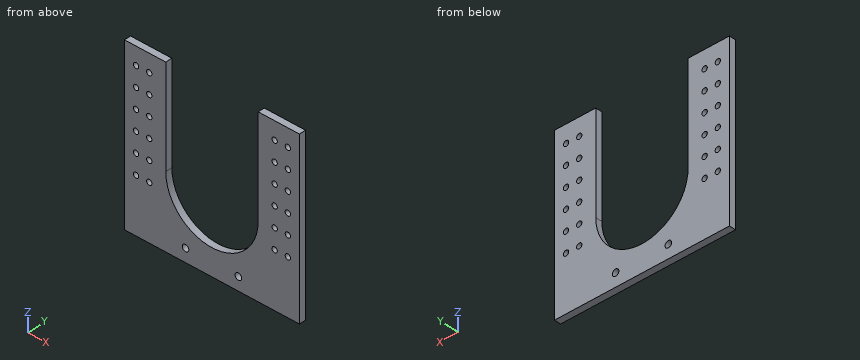
```python
from build123d import *

# Parameters (mm, degrees)
SKETCH1_W                        = 168.275
SKETCH1_H                        = 165.1
BOSS_EXTRUDE1_DEPTH              = 3.175
CUT_EXTRUDE1_REACH               = 120.042
SKETCH2_R                        = 44.45
F_1_4_0_25_DIAMETER_HOLE1_D      = 6.35
F_1_4_0_25_DIAMETER_HOLE1_DEPTH  = 25.4
F_1_4_0_25_DIAMETER_HOLE1_TIP    = 1.907732465
F_1_4_20_TAPPED_HOLE1_AT_2_COUNT = 2
F_1_4_20_TAPPED_HOLE1_AT_2_PITCH = 12.7
LPATTERN1_COUNT                  = 6
LPATTERN1_PITCH                  = 19.05


with BuildPart() as part:
    # Sketch1 → Boss-Extrude1 (new, symmetric)
    with BuildSketch(Plane(origin=(0, 0, 0), x_dir=(1, 0, 0), z_dir=(0, 1, 0))):
        Rectangle(SKETCH1_W, SKETCH1_H)
    extrude(amount=BOSS_EXTRUDE1_DEPTH, both=True)

    # Sketch2 → Cut-Extrude1 (cut, up to next)
    with BuildSketch(Plane(origin=(0, 3.175, 0), x_dir=(1, 0, 0), z_dir=(0, 1, 0)), mode=Mode.PRIVATE) as cut_extrude1_sk1:
        with Locations((0, 12.7)):
            Circle(SKETCH2_R)
    cut_extrude1_tool1 = extrude(cut_extrude1_sk1.sketch, amount=-CUT_EXTRUDE1_REACH, mode=Mode.PRIVATE) & part.part
    # Sketch2 → Cut-Extrude1 (cut, up to next)
    with BuildSketch(Plane(origin=(0, 3.175, 0), x_dir=(1, 0, 0), z_dir=(0, 1, 0)), mode=Mode.PRIVATE) as cut_extrude1_sk2:
        with BuildLine():
            Line((44.45, -82.55), (44.45, 12.7))
            ThreePointArc((44.45, 12.7), (0, -31.75), (-44.45, 12.7))
            Line((-44.45, 12.7), (-44.45, -82.55))
            Line((-44.45, -82.55), (44.45, -82.55))
        make_face()
    cut_extrude1_tool2 = extrude(cut_extrude1_sk2.sketch, amount=-CUT_EXTRUDE1_REACH, mode=Mode.PRIVATE) & part.part
    add(cut_extrude1_tool1.solids().sort_by_distance((0, 3.175, -12.7))[0], mode=Mode.SUBTRACT)
    add(cut_extrude1_tool2.solids().sort_by_distance((0, 3.175, 51.564855))[0], mode=Mode.SUBTRACT)

    # 1/4 (0.25) Diameter Hole1
    with Locations(Plane(origin=(0, 3.175, 0), x_dir=(1, 0, 0), z_dir=(0, 1, 0))):
        with Locations((-25.4, 69.85), (25.4, 69.85)):
            Hole(F_1_4_0_25_DIAMETER_HOLE1_D / 2, depth=F_1_4_0_25_DIAMETER_HOLE1_DEPTH)
            with Locations((0, 0, -(F_1_4_0_25_DIAMETER_HOLE1_DEPTH + F_1_4_0_25_DIAMETER_HOLE1_TIP / 2))):  # 118° drill point
                Cone(0, F_1_4_0_25_DIAMETER_HOLE1_D / 2, F_1_4_0_25_DIAMETER_HOLE1_TIP, mode=Mode.SUBTRACT)

    # Sketch10 → 1/4-20 Tapped Hole1 (revolve, cut)
    with BuildSketch(Plane(origin=(-73.025, 3.175, 65.603705108), x_dir=(0, 0, 1), z_dir=(1, 0, 0))):
        Polygon((0, 0), (0, 26.933816902), (2.5527, 25.4), (2.5527, 0), align=None)
    f_1_4_20_tapped_hole1 = revolve(axis=Axis((-73.025, 9.525, 65.603705108), (0, -1, 0)), mode=Mode.SUBTRACT)

    # 1/4-20 Tapped Hole1 at 2: 1/4-20 Tapped Hole1 ×2
    with Locations(*[(i * F_1_4_20_TAPPED_HOLE1_AT_2_PITCH, 0, 0) for i in range(1, F_1_4_20_TAPPED_HOLE1_AT_2_COUNT)]):
        add(f_1_4_20_tapped_hole1, mode=Mode.SUBTRACT)

    # LPattern1: 1/4-20 Tapped Hole1 ×6
    with Locations(*[(0, 0, -i * LPATTERN1_PITCH) for i in range(1, LPATTERN1_COUNT)]):
        add(f_1_4_20_tapped_hole1, mode=Mode.SUBTRACT)

    # LPattern1 copy 1 sketch → LPattern1 copy 1 (revolve, cut)
    with BuildSketch(Plane(origin=(-60.325, 3.175, 46.553705108), x_dir=(0, 0, 1), z_dir=(1, 0, 0))):
        Polygon((0, 0), (0, 26.933816902), (2.5527, 25.4), (2.5527, 0), align=None)
    revolve(axis=Axis((-60.325, 9.525, 46.553705108), (0, -1, 0)), mode=Mode.SUBTRACT)

    # LPattern1 copy 2 sketch → LPattern1 copy 2 (revolve, cut)
    with BuildSketch(Plane(origin=(-60.325, 3.175, 27.503705108), x_dir=(0, 0, 1), z_dir=(1, 0, 0))):
        Polygon((0, 0), (0, 26.933816902), (2.5527, 25.4), (2.5527, 0), align=None)
    revolve(axis=Axis((-60.325, 9.525, 27.503705108), (0, -1, 0)), mode=Mode.SUBTRACT)

    # LPattern1 copy 3 sketch → LPattern1 copy 3 (revolve, cut)
    with BuildSketch(Plane(origin=(-60.325, 3.175, 8.453705108), x_dir=(0, 0, 1), z_dir=(1, 0, 0))):
        Polygon((0, 0), (0, 26.933816902), (2.5527, 25.4), (2.5527, 0), align=None)
    revolve(axis=Axis((-60.325, 9.525, 8.453705108), (0, -1, 0)), mode=Mode.SUBTRACT)

    # LPattern1 copy 4 sketch → LPattern1 copy 4 (revolve, cut)
    with BuildSketch(Plane(origin=(-60.325, 3.175, -10.596294892), x_dir=(0, 0, 1), z_dir=(1, 0, 0))):
        Polygon((0, 0), (0, 26.933816902), (2.5527, 25.4), (2.5527, 0), align=None)
    revolve(axis=Axis((-60.325, 9.525, -10.596294892), (0, -1, 0)), mode=Mode.SUBTRACT)

    # LPattern1 copy 5 sketch → LPattern1 copy 5 (revolve, cut)
    with BuildSketch(Plane(origin=(-60.325, 3.175, -29.646294892), x_dir=(0, 0, 1), z_dir=(1, 0, 0))):
        Polygon((0, 0), (0, 26.933816902), (2.5527, 25.4), (2.5527, 0), align=None)
    revolve(axis=Axis((-60.325, 9.525, -29.646294892), (0, -1, 0)), mode=Mode.SUBTRACT)

    # Mirror1: 1/4-20 Tapped Hole1 across plane
    add(f_1_4_20_tapped_hole1.mirror(Plane(origin=(0, 0, 0), x_dir=(0, 0, 1), z_dir=(1, 0, 0))), mode=Mode.SUBTRACT)

    # Mirror1 copy 1 sketch → Mirror1 copy 1 (revolve, cut)
    with BuildSketch(Plane(origin=(60.325, 3.175, 65.603705108), x_dir=(0, 0, 1), z_dir=(-1, 0, 0))):
        Polygon((0, 0), (0, -26.933816902), (2.5527, -25.4), (2.5527, 0), align=None)
    revolve(axis=Axis((60.325, 9.525, 65.603705108), (0, 1, 0)), mode=Mode.SUBTRACT)

    # Mirror1 copy 2 sketch → Mirror1 copy 2 (revolve, cut)
    with BuildSketch(Plane(origin=(73.025, 3.175, 46.553705108), x_dir=(0, 0, 1), z_dir=(-1, 0, 0))):
        Polygon((0, 0), (0, -26.933816902), (2.5527, -25.4), (2.5527, 0), align=None)
    revolve(axis=Axis((73.025, 9.525, 46.553705108), (0, 1, 0)), mode=Mode.SUBTRACT)

    # Mirror1 copy 3 sketch → Mirror1 copy 3 (revolve, cut)
    with BuildSketch(Plane(origin=(73.025, 3.175, 27.503705108), x_dir=(0, 0, 1), z_dir=(-1, 0, 0))):
        Polygon((0, 0), (0, -26.933816902), (2.5527, -25.4), (2.5527, 0), align=None)
    revolve(axis=Axis((73.025, 9.525, 27.503705108), (0, 1, 0)), mode=Mode.SUBTRACT)

    # Mirror1 copy 4 sketch → Mirror1 copy 4 (revolve, cut)
    with BuildSketch(Plane(origin=(73.025, 3.175, 8.453705108), x_dir=(0, 0, 1), z_dir=(-1, 0, 0))):
        Polygon((0, 0), (0, -26.933816902), (2.5527, -25.4), (2.5527, 0), align=None)
    revolve(axis=Axis((73.025, 9.525, 8.453705108), (0, 1, 0)), mode=Mode.SUBTRACT)

    # Mirror1 copy 5 sketch → Mirror1 copy 5 (revolve, cut)
    with BuildSketch(Plane(origin=(73.025, 3.175, -10.596294892), x_dir=(0, 0, 1), z_dir=(-1, 0, 0))):
        Polygon((0, 0), (0, -26.933816902), (2.5527, -25.4), (2.5527, 0), align=None)
    revolve(axis=Axis((73.025, 9.525, -10.596294892), (0, 1, 0)), mode=Mode.SUBTRACT)

    # Mirror1 copy 6 sketch → Mirror1 copy 6 (revolve, cut)
    with BuildSketch(Plane(origin=(73.025, 3.175, -29.646294892), x_dir=(0, 0, 1), z_dir=(-1, 0, 0))):
        Polygon((0, 0), (0, -26.933816902), (2.5527, -25.4), (2.5527, 0), align=None)
    revolve(axis=Axis((73.025, 9.525, -29.646294892), (0, 1, 0)), mode=Mode.SUBTRACT)

    # Mirror1 copy 7 sketch → Mirror1 copy 7 (revolve, cut)
    with BuildSketch(Plane(origin=(60.325, 3.175, 46.553705108), x_dir=(0, 0, 1), z_dir=(-1, 0, 0))):
        Polygon((0, 0), (0, -26.933816902), (2.5527, -25.4), (2.5527, 0), align=None)
    revolve(axis=Axis((60.325, 9.525, 46.553705108), (0, 1, 0)), mode=Mode.SUBTRACT)

    # Mirror1 copy 8 sketch → Mirror1 copy 8 (revolve, cut)
    with BuildSketch(Plane(origin=(60.325, 3.175, 27.503705108), x_dir=(0, 0, 1), z_dir=(-1, 0, 0))):
        Polygon((0, 0), (0, -26.933816902), (2.5527, -25.4), (2.5527, 0), align=None)
    revolve(axis=Axis((60.325, 9.525, 27.503705108), (0, 1, 0)), mode=Mode.SUBTRACT)

    # Mirror1 copy 9 sketch → Mirror1 copy 9 (revolve, cut)
    with BuildSketch(Plane(origin=(60.325, 3.175, 8.453705108), x_dir=(0, 0, 1), z_dir=(-1, 0, 0))):
        Polygon((0, 0), (0, -26.933816902), (2.5527, -25.4), (2.5527, 0), align=None)
    revolve(axis=Axis((60.325, 9.525, 8.453705108), (0, 1, 0)), mode=Mode.SUBTRACT)

    # Mirror1 copy 10 sketch → Mirror1 copy 10 (revolve, cut)
    with BuildSketch(Plane(origin=(60.325, 3.175, -10.596294892), x_dir=(0, 0, 1), z_dir=(-1, 0, 0))):
        Polygon((0, 0), (0, -26.933816902), (2.5527, -25.4), (2.5527, 0), align=None)
    revolve(axis=Axis((60.325, 9.525, -10.596294892), (0, 1, 0)), mode=Mode.SUBTRACT)

    # Mirror1 copy 11 sketch → Mirror1 copy 11 (revolve, cut)
    with BuildSketch(Plane(origin=(60.325, 3.175, -29.646294892), x_dir=(0, 0, 1), z_dir=(-1, 0, 0))):
        Polygon((0, 0), (0, -26.933816902), (2.5527, -25.4), (2.5527, 0), align=None)
    revolve(axis=Axis((60.325, 9.525, -29.646294892), (0, 1, 0)), mode=Mode.SUBTRACT)


solid = part.part
```
Input: part model. Units: mm. Frame: model coordinates. Round coordinates to 2 decimals unless told otherwise and drop trailing zeros. Loops run counter-clockwise (first coordinate to the right, second up) from the corner with the lowest first, then second, coordinate; pieces in that order, holes last. Notation, with made-up numbers: (87, -13.5) -> (117, -13.5) arc R30 cw to (117, 20.5) -> close; hole circle Ø9 at (40.5, -33.5). An arc over 180 degrees is marked (long way). One line per item, written item: value.
(1) Pin query (flat end, axial travel): pin 1 (4.5 mm diameter, centred on x = 60.32, z = -10.6, fed in from -Y). Return the tip coordinate at first contact, or that it passes through.
Geometry check:
pin 1: through
(2) Section C-C (x = 25.4). Return the cut outline in (y, z) (3 decimals), plus the area to 3 significant figures.
Geometry check:
outline: (-3.175, -82.55) -> (3.175, -82.55) -> (3.175, -73.025) -> (-3.175, -73.025) -> close; (-3.175, -66.675) -> (3.175, -66.675) -> (3.175, -49.178) -> (-3.175, -49.178) -> close
area: 172 mm2
(3) Section B-B (y = 1.5). Give the number of separate pieces and of enclosed holes in the cut face, plus the area to 3 significant figures.
Geometry check:
separate pieces: 1
enclosed holes: 26
area: 15,700 mm2
(4) Section A-A (z = -69.85). Return the cut outline in (x, y) (1 decimal).
Geometry check:
outline: (-84.1, -3.2) -> (-28.6, -3.2) -> (-28.6, 3.2) -> (-84.1, 3.2) -> close; (-22.2, -3.2) -> (22.2, -3.2) -> (22.2, 3.2) -> (-22.2, 3.2) -> close; (28.6, -3.2) -> (84.1, -3.2) -> (84.1, 3.2) -> (28.6, 3.2) -> close
(5) Section D-D (x = 0). Return the cut outline in (y, z) (3 decimals), plus the area to 3 significant figures.
Geometry check:
outline: (-3.175, -82.55) -> (3.175, -82.55) -> (3.175, -57.15) -> (-3.175, -57.15) -> close
area: 161 mm2
(6) Material intervals for line 1 (X direction, y = -2.25, z = 27.5); line 2 (X direction, y = 1, z = 61.5); line 3 (X direction, y = 0, z = 9.5), sorted ascending. Write a range as [from, to].
Geometry check:
line 1: [-84.14, -75.58], [-70.47, -62.88], [-57.77, -44.45], [44.45, 57.77], [62.88, 70.47], [75.58, 84.14]
line 2: [-84.14, -44.45], [44.45, 84.14]
line 3: [-84.14, -75.35], [-70.7, -62.65], [-58, -44.45], [44.45, 58], [62.65, 70.7], [75.35, 84.14]
